Can you work these out from the drawing? Everything is in mm from the part's minimum corner. A direction names the side the tool comes from. Give positions to 0.01 mm unless a question says otherwise; leave off trailing zeros. Loops run counter-clockwise (first coordinate to the right, second up) from the corner with the lowest first, then second, coordinate; pieces in that order, holes last. Notation, with made-up numbers: (-12, 54.5) -> (7, 54.5) arc R26 cw to (7, 72.5) -> close; hole circle Ø6 at (53, 86.25). An arc over 180 degrees is marked (long way). Write item = value, one per line. Start each with the question number.
1) I want a section at B-B (y = 26). List the corners of the cut face in (x, z) for me.
2) I want a section at A-A (x = 19.5). List the corners of the cut face in (y, z) for me.
3) I want a section at C-C (z = 5.5). List the corners of the cut face in (x, y) for me.
4) I want a section at D-D (x = 36.5). List the corners of the cut face in (y, z) for me.
5) On a 3-axis mill with a long thin cutter (end or side, diameter ignored), from which of +Z, -Z, +X, -X, +Y, -Y can I reach the whole of each face in a straight line? I mean the marked faces 3 and 4. Say none if no direction works.
6) I'm going to push a flat-ended pin straight in: pin 1 Ø0.9 at (x, z) = (22, 1.87) entering from +Y. Where does the tip first touch, or does it pass through?
7) I need wall thicknesses on probe 1 along Z at (x, y) = (40, 22); probe 2 along Z at (x, y) = (21.5, 30) (1 decimal); probe 3 along Y at (x, z) = (24.5, 5.75). Which ranges of each line are inside material? Lowest first, please. Write a range as from..to.
8) If we mould it in two halves opening along X, with no side actions, what happens to the marked faces 1 and 2? For each: +X half, -X half, draft (parallel to the pull), parting line (faces both ways), or undercut.
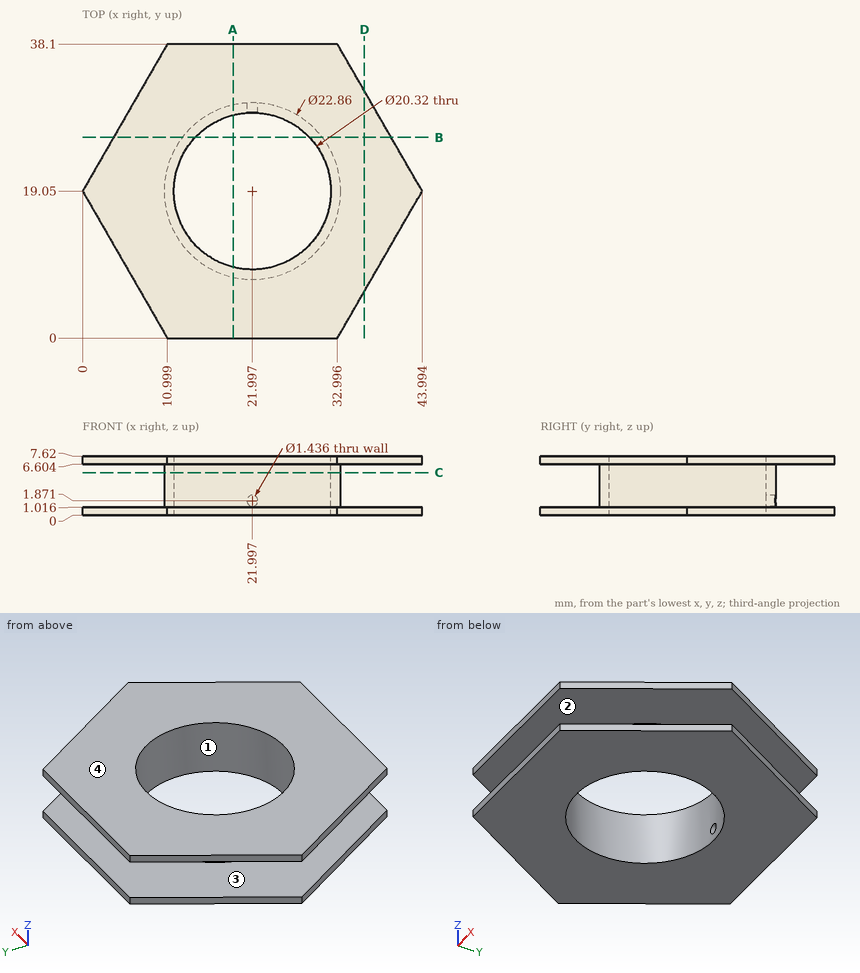
Answer list:
q1.outline = (4.01, 0) -> (14.59, 0) -> (14.59, 7.62) -> (4.01, 7.62) -> (4.01, 6.6) -> (12.92, 6.6) -> (12.92, 1.02) -> (4.01, 1.02) -> close; (29.41, 0) -> (39.98, 0) -> (39.98, 1.02) -> (31.07, 1.02) -> (31.07, 6.6) -> (39.98, 6.6) -> (39.98, 7.62) -> (29.41, 7.62) -> close
q2.outline = (0, 0) -> (9.2, 0) -> (9.2, 7.62) -> (0, 7.62) -> (0, 6.6) -> (7.9, 6.6) -> (7.9, 1.02) -> (0, 1.02) -> close; (28.9, 0) -> (38.1, 0) -> (38.1, 1.02) -> (30.2, 1.02) -> (30.2, 6.6) -> (38.1, 6.6) -> (38.1, 7.62) -> (28.9, 7.62) -> close
q3.outline = circle Ø22.86 at (22, 19.05); hole circle Ø20.32 at (22, 19.05)
q4.outline = (6.07, 0) -> (32.03, 0) -> (32.03, 1.02) -> (6.07, 1.02) -> close; (6.07, 6.6) -> (32.03, 6.6) -> (32.03, 7.62) -> (6.07, 7.62) -> close
q5.face_3 = none
q5.face_4 = +Z, +X, -X, +Y, -Y
q6.pin_1 = 8.9
q7.probe_1 = 0..1.02, 6.6..7.62
q7.probe_2 = 0..1.4, 2.4..7.6
q7.probe_3 = 7.9..9.2, 28.9..30.2
q8.face_1 = undercut
q8.face_2 = draft
